```python
from build123d import *

# Parameters (mm, degrees)
EXTRUDE1_DEPTH     = 16.51
CUT_EXTRUDE1_DEPTH = 10.16
EXTRUDE2_START     = -3.302
SKETCH2_W          = 1.016
SKETCH2_H          = 1.016
EXTRUDE2_DEPTH     = 13.97
LPATTERN1_COUNT    = 3
LPATTERN1_PITCH    = 5.08


with BuildPart() as part:
    # Sketch1 → Extrude1 (new body)
    with BuildSketch(Plane(origin=(3.175, 0, 0), x_dir=(0, 0, -1), z_dir=(1, 0, 0))):
        Polygon((-3.9751, 0), (-3.9751, 9.906), (-4.4069, 9.906), (-4.4069, 10.668), (-3.673665158, 11.938), (3.9751, 11.938), (3.9751, 0), align=None)
    extrude(amount=-EXTRUDE1_DEPTH)

    # Sketch3 → Cut-Extrude1 (cut)
    with BuildSketch(Plane(origin=(0, 11.938, 0), x_dir=(1, 0, 0), z_dir=(0, 1, 0))):
        with BuildLine():
            Line((-2.5654, 1.800881758), (-2.5654, -2.54))
            Line((-2.5654, -2.54), (2.5654, -2.54))
            Line((2.5654, -2.54), (2.5654, 1.800881758))
            ThreePointArc((2.5654, 1.800881758), (0, 2.794), (-2.5654, 1.800881758))
        make_face()
    cut_extrude1 = extrude(amount=-CUT_EXTRUDE1_DEPTH, mode=Mode.SUBTRACT)

    # Sketch2 → Extrude2 (add)
    with BuildSketch(Plane(origin=(0, 0, 0), x_dir=(1, 0, 0), z_dir=(0, 1, 0)).offset(EXTRUDE2_START)):
        Rectangle(SKETCH2_W, SKETCH2_H)
    extrude2 = extrude(amount=EXTRUDE2_DEPTH)

    # LPattern1: Cut-Extrude1, Extrude2 ×3
    with Locations(*[(-i * LPATTERN1_PITCH, 0, 0) for i in range(1, LPATTERN1_COUNT)]):
        add(cut_extrude1, mode=Mode.SUBTRACT)
        add(extrude2)


solid = part.part
```
Can you work these out from the model? Positions are in its coordinate system, mm. A direction names the side the tool comes from. Round coordinates to 2 decimals unless told otherwise and drop trailing zeros. Loops run counter-clockwise (first coordinate to the right, second up) from the corner with the lowest first, then second, coordinate; pieces in that order, holes last. Notation, with made-up numbers: M -38,9 L -23,9 A12 ccw -23,29 Z; hole C -15.75,80.25 d9. An arc over 180 degrees is marked long. Write item = value, one per line. Start each with the question number.
(1) Suppose I cut it at A-A on y = 3.75. Write out the boundary of the cut face in (x, z) (3 decimals), plus the area to 3 significant figures.
(2) If we mould it in two halves opening along Z, with no side actions, what happens to faces 5 (the face through (-10, -3.302, 0)), 6 (the face through (-12.725, 7, 0)), 7 (the face through (-5, 6, -0.508)), 8 (the face through (-5, -2, -0.508))? For each: released by +Z, released by -Z, zero draft, split by the parting line, or undercut.
(3) Suppose I cut it at B-B on y = -0.5. Write out the boundary of the cut face in (x, z).
(4) Suppose I cut it at D-D on x = 1.75. Write out the boundary of the cut face in (y, z), plus the area to 3 significant figures.
(5) Suppose I cut it at C-C on z = 2.25. Write out the boundary of the cut face in (x, y) (3 decimals).
(6) I'm going to push flat-ended pins straight in: P1, Ø1.1, axis at x = 0, y = 6.5, coming from the +Z side; P2, Ø0.5, axis at y = -1.5, z = 0, coming from the +X side; P3, Ø2.5, axis at x = -7.5, z = 0.5, coming from the -Y side; P4, Ø4.5, axis at x = -8, z = -0.5, coming from the +Y side. Where does each tip first touch, or does it pass through?
(7) Which directions (+Z, -Z, +X, -X, +Y, -Y) give clear straight access to the entire face, cutting with the end or side of a thin tool? Please do faces 1 (the face through (-5.588, -2, 0)), 2 (the face through (-6, 11.938, -3)), 3 (the face through (-5, 7, 2.54)), 4 (the face through (-10, -2, 0.508)).
(8) I need wall thicknesses on line 1 along X through (y, z) = (8.5, 0) (3 decimals); line 2 along X through (y, z) = (4.75, 2.5) (3 decimals); line 3 along X through (y, z) = (5.75, -2) (3 decimals). Which ranges of each line are inside material? Lowest first, please.
Answer block:
q1.outline = M -13.335,-3.975 L 3.175,-3.975 L 3.175,3.975 L -13.335,3.975 Z; M -10.668,-0.508 L -9.652,-0.508 L -9.652,0.508 L -10.668,0.508 Z; M -5.588,-0.508 L -4.572,-0.508 L -4.572,0.508 L -5.588,0.508 Z; M -0.508,-0.508 L 0.508,-0.508 L 0.508,0.508 L -0.508,0.508 Z; hole M -12.725,-1.801 A3.81 ccw -7.62,-1.824 A3.81 ccw -2.54,-1.824 A3.81 ccw 2.565,-1.801 L 2.565,2.54 L -12.725,2.54 Z
q1.area = 57.5 mm²
q2.face_5 = zero draft
q2.face_6 = undercut
q2.face_7 = undercut
q2.face_8 = released by -Z
q3.outline = M -10.67,-0.51 L -9.65,-0.51 L -9.65,0.51 L -10.67,0.51 Z; M -5.59,-0.51 L -4.57,-0.51 L -4.57,0.51 L -5.59,0.51 Z; M -0.51,-0.51 L 0.51,-0.51 L 0.51,0.51 L -0.51,0.51 Z
q4.outline = M 0,-3.98 L 11.94,-3.98 L 11.94,-2.37 L 1.78,-2.37 L 1.78,2.54 L 11.94,2.54 L 11.94,3.67 L 10.67,4.41 L 9.91,4.41 L 9.91,3.98 L 0,3.98 Z
q4.area = 45.5 mm²
q5.outline = M -13.335,0 L 3.175,0 L 3.175,11.938 L 2.565,11.938 L 2.565,1.778 L -12.725,1.778 L -12.725,11.938 L -13.335,11.938 Z
q6.P1 = 3.98
q6.P2 = 0.51
q6.P3 = 0
q6.P4 = 11.94
q7.face_1 = +Z, -Z, -Y
q7.face_2 = +Z, -Z, +X, -X, +Y
q7.face_3 = +Y
q7.face_4 = +Z, +X, -X, -Y
q8.line_1 = -13.335 to -12.725, -10.668 to -9.652, -5.588 to -4.572, -0.508 to 0.508, 2.565 to 3.175
q8.line_2 = -13.335 to -12.725, 2.565 to 3.175
q8.line_3 = -13.335 to -12.488, -7.832 to -7.408, -2.752 to -2.328, 2.328 to 3.175
